Model file for the job. Use its own axes, mm. Face numbers are marked on the shaded views. A direction names the side the tool comes from. Coordinates: 2 decimals unless noted, no trailing zeros. Loops run counter-clockwise (first coordinate to the right, second up) from the corner with the lowest first, then second, coordinate; pieces in that order, holes last. Notation, with made-up numbers: (30, -36) -> (47, -36) arc R27 cw to (47, -8) -> close; hole circle Ø1 at (21.5, -18). An arc over 180 degrees is marked (long way). Use one line per item in the form item = value.
```python
from build123d import *

# Parameters (mm, degrees)
SKETCH_1_W            = 164.9
SKETCH_1_H            = 100
EXTRUDE_319_DEPTH     = 6
SKETCH_2_W            = 156.7
SKETCH_2_H            = 89.1
CUT_EXTRUDE_496_DEPTH = 0.1
SKETCH_4_W            = 35.5
SKETCH_4_H            = 0.3
EXTRUDE_2_DEPTH       = 80.15
CUT_EXTRUDE_4_DEPTH   = 155.144566884
SKETCH_6_W            = 25.5
SKETCH_6_H            = 3.8
CUT_EXTRUDE_5_DEPTH   = 0.05


with BuildPart() as part:
    # 草图1 → Extrude 319 (new body)
    with BuildSketch(Plane.XY):
        Rectangle(SKETCH_1_W, SKETCH_1_H)
    extrude(amount=EXTRUDE_319_DEPTH)

    # 草图2 → Cut-Extrude 496 (cut)
    with BuildSketch(Plane.XY):
        with Locations((1.39, 1.88)):
            Rectangle(SKETCH_2_W, SKETCH_2_H)
    extrude(amount=CUT_EXTRUDE_496_DEPTH, mode=Mode.SUBTRACT)

    # 草图4 → 凸台-拉伸2 (add)
    with BuildSketch(Plane.XZ.offset(50)):
        with Locations((-1.5, 5)):
            Rectangle(SKETCH_4_W, SKETCH_4_H)
    extrude(amount=EXTRUDE_2_DEPTH)

    # 草图5 → 切除-拉伸4 (cut, through all)
    with BuildSketch(Plane(origin=(0, 0, 4.85), x_dir=(-1, 0, 0), z_dir=(0, 0, -1))):
        Polygon((-16.25, -130.15), (-11.25, -130.15), (-11.25, -76.987179315), (-16.25, -64.867086026), align=None)
        Polygon((19.25, -130.15), (14.25, -130.15), (14.25, -67.739612604), (19.25, -54.255364134), align=None)
    extrude(amount=-CUT_EXTRUDE_4_DEPTH, mode=Mode.SUBTRACT)

    # 草图6 → 切除-拉伸5 (cut)
    with BuildSketch(Plane(origin=(0, 0, 4.85), x_dir=(-1, 0, 0), z_dir=(0, 0, -1))):
        with Locations((1.5, -128.25)):
            Rectangle(SKETCH_6_W, SKETCH_6_H)
    extrude(amount=-CUT_EXTRUDE_5_DEPTH, mode=Mode.SUBTRACT)


solid = part.part
```
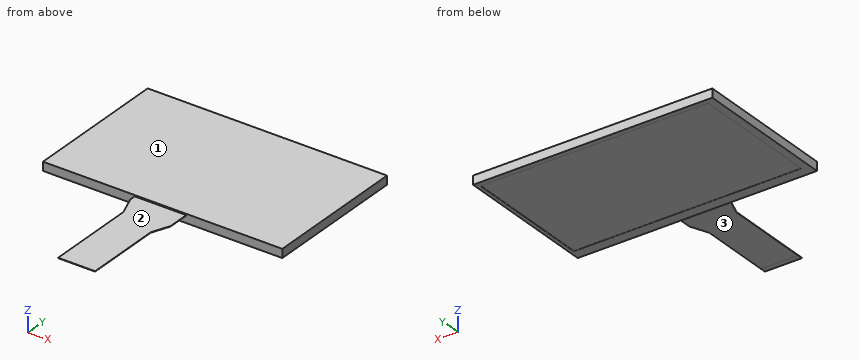
Q1. Band-saw the part on B-B, the plane x = 22.5. Write the cut outline in (y, z).
Result:
outline = (-50, 0) -> (-42.67, 0) -> (-42.67, 0.1) -> (46.43, 0.1) -> (46.43, 0) -> (50, 0) -> (50, 6) -> (-50, 6) -> close
Q2. Wall check: line 1 along Y through (x, z) = (18, 3.4); line 2 along Z through (x, y) = (6, -11); line 3 along Z through (x, y) = (3.5, -108). Give the ranges that are in metal, low to high.
Result:
line_1 = -50 to 50
line_2 = 0.1 to 6
line_3 = 4.85 to 5.15
Q3. Which spindle directions (+Z, -Z, +X, -X, +Y, -Y) get a long thin tool onto all of the face, cutting with end or side? Do the marked faces 1, 2 and 3. Say none if no direction does.
Result:
face_1 = +Z, +X, -X, +Y, -Y
face_2 = +Z, +X, -X, -Y
face_3 = -Z, +X, -X, -Y
Q4. Band-saw the part on A-A, the plane y = 9.5. Write the cut outline in (x, z), and give its area (3 significant figures).
Result:
outline = (-82.45, 0) -> (-76.96, 0) -> (-76.96, 0.1) -> (79.74, 0.1) -> (79.74, 0) -> (82.45, 0) -> (82.45, 6) -> (-82.45, 6) -> close
area = 974 mm2
Q5. Pin check, flat tips, straight feed: pin 1 Ø1.5 at (x, z) = (18, 1) entering from -Y; pin 2 Ø3 at (x, y) = (-5.5, -128) entering from -Z; pin 3 Ø18 at (x, y) = (7, -103) entering from -Z. Stop position of each tip, or through.
Result:
pin_1 = -50
pin_2 = 4.9
pin_3 = 4.85
Q6. Band-saw the part on D-D, the plane y = -111.5. Write the cut outline in (x, z).
Result:
outline = (-14.25, 4.85) -> (11.25, 4.85) -> (11.25, 5.15) -> (-14.25, 5.15) -> close
Q7. Band-saw the part on C-C, the plane z = 2.3. Write the cut outline in (x, y), and give its area (3 significant figures).
Result:
outline = (-82.45, -50) -> (82.45, -50) -> (82.45, 50) -> (-82.45, 50) -> close
area = 16,500 mm2
